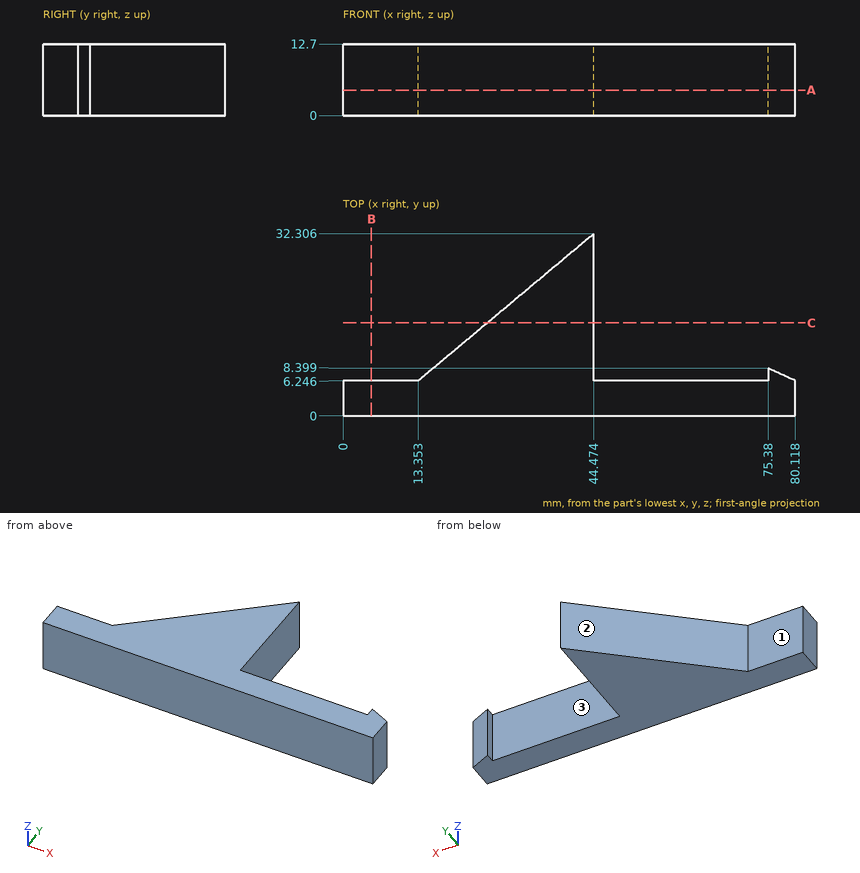
Could you check a few things on this drawing? It's one solid part, dimensions in mm from its lowest x, y, z. Coordinates: 2 decimals unless noted, no trailing zeros. Order: outer loops, then holes, each group sorted by start corner. A loop starts at its lowest first (then second) coordinate and runs counter-clockwise, first axis right, second up. Notation, with made-up numbers: (-39.75, 69) -> (-11.75, 69) arc R6 ccw to (-11.75, 73) -> close; hole circle Ø11 at (-31.75, 79.25). An arc over 180 degrees is marked (long way). One line per item, written item: value. Start each with the question number.
1) Imagine slicing it at B-B on x = 5. List the corners of the cut face in (y, z) for me (1 decimal).
2) Imagine slicing it at A-A on z = 4.5. List the corners of the cut face in (x, y) for me (1 decimal), plus the area to 3 significant figures.
3) I'm going to push flat-ended pins straight in: pin 1 (0.6 mm diameter, centred on y = 8, z = 3.5, fed in from -X); pin 2 (2 mm diameter, centred on y = 13.5, z = 2.5, fed in from +X); pin 3 (4 mm diameter, centred on x = 8, z = 6.5, fed in from +Y); pin 4 (8 mm diameter, centred on x = 64, y = 11.5, fed in from +Z). Where does each tip first touch, or does it pass through?
4) If I drill on L1, parallel to Y at x = 12.5, z = 10.5 (1 decimal); L2, parallel to Y at x = 41.5, z = 8.75 (1 decimal); L3, parallel to X at y = 19, z = 11.25 (1 decimal), over which ranges is the centre line in solid material (lowest first)? Write a range as [from, to].
5) Imagine slicing it at C-C on y = 16.5. List the corners of the cut face in (x, z) for me, plus the area to 3 significant figures.
6) We'd pull the mould along X, two halves only. Please class the marked faces 1, 2 and 3: +X half, -X half, draft (parallel to the pull), parting line (faces both ways), or undercut.
Answer list:
1. outline: (0, 0) -> (6.2, 0) -> (6.2, 12.7) -> (0, 12.7) -> close
2. outline: (0, 0) -> (80.1, 0) -> (80.1, 6.2) -> (75.4, 8.4) -> (75.4, 6.2) -> (44.5, 6.2) -> (44.5, 32.3) -> (13.4, 6.2) -> (0, 6.2) -> close
2. area: 911 mm2
3. pin 1: stops at x = 15.09
3. pin 2: stops at x = 44.47
3. pin 3: stops at y = 6.25
3. pin 4: passes through
4. L1: y = [0, 6.2]
4. L2: y = [0, 29.8]
4. L3: x = [28.6, 44.5]
5. outline: (25.6, 0) -> (44.47, 0) -> (44.47, 12.7) -> (25.6, 12.7) -> close
5. area: 240 mm2
6. face 1: draft
6. face 2: -X half
6. face 3: undercut
